Read the model definition and answer for the solid it produces. Units are mm, in the model's axes. Face numbers are marked on the shaded views. A direction names the side the tool comes from. Round coordinates to 2 decimals unless told otherwise and drop trailing zeros. Loops run counter-clockwise (first coordinate to the right, second up) from the corner with the lowest first, then second, coordinate; pieces in that order, holes last. Notation, with made-up numbers: M 1.5,26 L 33.5,26 A34 ccw 33.5,63 Z; hole C -28,55.25 d2. An arc over 180 degrees is marked long. Write each question's results on one line, items separated by ' | '.
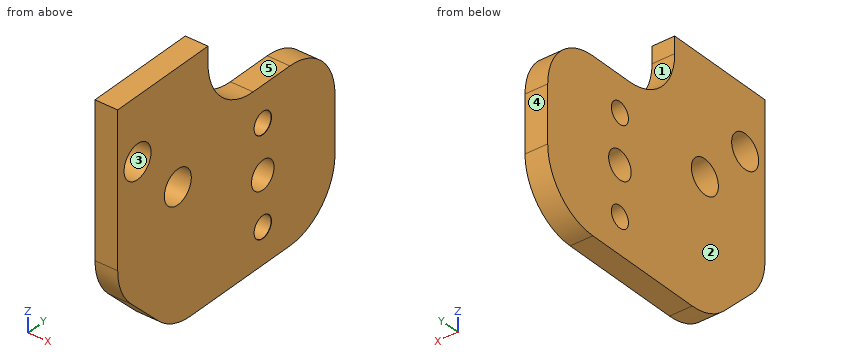
from build123d import *

# Parameters (mm, degrees)
SKETCH1_W                      = 19.05
SKETCH1_H                      = 30.5721766
BOSS_EXTRUDE1_DEPTH            = 2.54
SKETCH2_R                      = 1.5875
CUT_EXTRUDE1_DEPTH             = 33.122191816
M2_CLEARANCE_HOLE1_D           = 2.4
M2_CLEARANCE_HOLE1_DEPTH       = 12.0000014
M2_CLEARANCE_HOLE1_CSINK_D     = 2.45
M2_CLEARANCE_HOLE1_CSINK_ANGLE = 90
M2_CLEARANCE_HOLE1_TIP         = 0.721032743
SKETCH6_W                      = 8.2193384
SKETCH6_H                      = 12.7
BOSS_EXTRUDE2_DEPTH            = 2.54
CHAMFER1_SIZE                  = 7.62
FILLET2_R                      = 6.35
F_6_CLEARANCE_HOLE1_D          = 3.7973


with BuildPart() as part:
    # Sketch1 → Boss-Extrude1 (new body)
    with BuildSketch(Plane(origin=(0, 0, 0), x_dir=(0, 0, -1), z_dir=(1, 0, 0))):
        with Locations((0, 15.2860883)):
            Rectangle(SKETCH1_W, SKETCH1_H)
    extrude(amount=BOSS_EXTRUDE1_DEPTH)

    # Sketch2 → Cut-Extrude1 (cut, through all)
    with BuildSketch(Plane(origin=(2.54, 0, 0), x_dir=(0, 0, -1), z_dir=(1, 0, 0))):
        with Locations((0, 20.4121766)):
            Circle(SKETCH2_R)
    extrude(amount=-CUT_EXTRUDE1_DEPTH, mode=Mode.SUBTRACT)

    # M2 Clearance Hole1
    with Locations(Plane(origin=(2.54, 0, 0), x_dir=(0, 0, -1), z_dir=(1, 0, 0))):
        with Locations((-5.5, 20.4121766), (5.5, 20.4121766)):
            CounterSinkHole(M2_CLEARANCE_HOLE1_D / 2, M2_CLEARANCE_HOLE1_CSINK_D / 2, depth=M2_CLEARANCE_HOLE1_DEPTH, counter_sink_angle=M2_CLEARANCE_HOLE1_CSINK_ANGLE)
            with Locations((0, 0, -(M2_CLEARANCE_HOLE1_DEPTH + M2_CLEARANCE_HOLE1_TIP / 2))):  # 118° drill point
                Cone(0, M2_CLEARANCE_HOLE1_D / 2, M2_CLEARANCE_HOLE1_TIP, mode=Mode.SUBTRACT)

    # Sketch6 → Boss-Extrude2 (add)
    with BuildSketch(Plane(origin=(0, 0, 0), x_dir=(0, 0, -1), z_dir=(1, 0, 0))):
        with Locations((-13.6346692, 6.35)):
            Rectangle(SKETCH6_W, SKETCH6_H)
    extrude(amount=BOSS_EXTRUDE2_DEPTH)

    # Chamfer1
    chamfer1_edges = [part.edges().sort_by_distance(p)[0] for p in [
        (1.27, 0, -9.525),
    ]]
    chamfer(chamfer1_edges, length=CHAMFER1_SIZE)

    # Fillet2
    fillet2_edges = [part.edges().sort_by_distance(p)[0] for p in [
        (1.27, 12.7, 9.525),
        (1.27, 7.62, -9.525),
        (1.27, 0, -1.905),
        (1.27, 30.5721766, 9.525),
        (1.27, 30.5721766, -9.525),
    ]]
    fillet(fillet2_edges, radius=FILLET2_R)

    # #6 Clearance Hole1 (through all)
    with Locations(Plane.ZY):
        with Locations((10.7847384, 2.794), (5.0951384, 8.4582)):
            Hole(F_6_CLEARANCE_HOLE1_D / 2)


solid = part.part
Item 1: Flat-ended cylindrical pins translate along their axes: pin 1 (6 mm diameter, centred on y = 8.46, z = 5.1, fed in from -X); pin 2 (1.5 mm diameter, centred on x = 1.5, z = 16.5, fed in from +Y); pin 3 (1.3 mm diameter, centred on x = 1.5, y = 21, fed in from +Z) (3 decimals). Find the tip coordinate at first contact, or state that the pin passes through.
Outcome:
pin 1: stops at x = 0 | pin 2: stops at y = 12.7 | pin 3: stops at z = 9.525
Item 2: The part is cut by section B-B (x = 1.9). State how many separate pieces and enclosed holes the cut face has, plus the area to 3 significant figures.
Outcome:
separate pieces: 1 | enclosed holes: 5 | area: 608 mm2
Item 3: Straight lines are drawn through the part: line 1 (Z direction, x = 0.45, y = 21.5) (3 decimals); line 2 (Z direction, x = 0.65, y = 29.5); line 3 (Z direction, x = 1.75, y = 23.5) (3 decimals). For each, find the intervals that lie inside material, in ascending order.
Outcome:
line 1: z = -9.525 to -6.007, -4.993 to -1.156, 1.156 to 4.993, 6.007 to 9.525 | line 2: z = -6.71 to 6.71 | line 3: z = -9.525 to 9.525
Item 4: For the marked faces 4 and 5, determine the directions among +Z, -Z, +X, -X, +Y, -Y from which every point of the face is accessible in a straight line to the end or side of a thin tool.
Outcome:
face 4: +Z, -Z, +X, -X, +Y | face 5: +Z, +X, -X, +Y
Item 5: The part is cut by section A-A (z = -5.5). Determine the outline of the cut face in (x, y) (3 decimals).
Outcome:
outline: M 0,3.595 L 2.54,3.595 L 2.54,19.187 L 2.515,19.212 L 0,19.212 Z; M 0,21.612 L 2.515,21.612 L 2.54,21.637 L 2.54,30.131 L 0,30.131 Z
Item 6: The part is cut by section D-D (y = 23.5). Determine the outline of the cut face in (x, z) (3 decimals), plus the area to 3 significant figures.
Outcome:
outline: M 0,-9.525 L 2.54,-9.525 L 2.54,9.525 L 0,9.525 Z | area: 48.4 mm2
Item 7: The mould has two halves that part along Z. Classify the marked faces 1, 2 and 3: pulls with the +Z half, pulls with the -Z half, needs draft (parallel to the pull), parting line crosses it, or undercut.
Outcome:
face 1: pulls with the +Z half | face 2: needs draft | face 3: undercut
Item 8: The part is cut by section C-C (z = 5.5). Determine the outline of the cut face in (x, y) (3 decimals).
Outcome:
outline: M 0,0 L 2.54,0 L 2.54,6.603 L 0,6.603 Z; M 0,10.313 L 2.54,10.313 L 2.54,19.187 L 2.515,19.212 L 0,19.212 Z; M 0,21.612 L 2.515,21.612 L 2.54,21.637 L 2.54,30.131 L 0,30.131 Z
